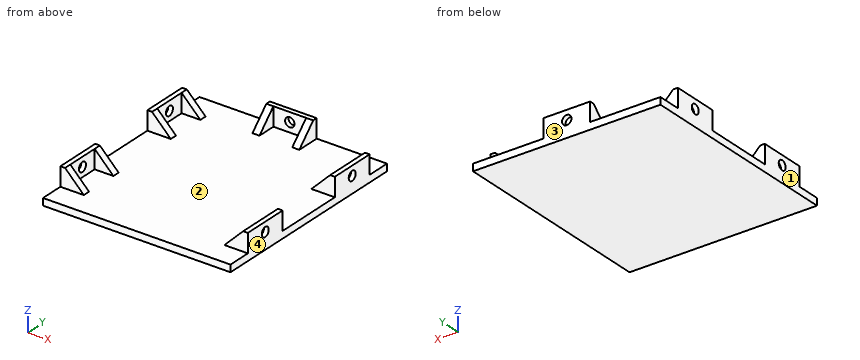
```python
from build123d import *

# Parameters (mm, degrees)
SKETCH1_W               = 80
SKETCH1_H               = 90
BOSS_EXTRUDE1_DEPTH     = 3
BOSS_EXTRUDE2_DEPTH     = 8
CUT_EXTRUDE1_DEPTH      = 114.670576668
SKETCH6_R               = 2
CUT_EXTRUDE3_DEPTH      = 25
MIRROR5_COPY_1_DEPTH    = 8
MIRROR5_COPY_2_DEPTH    = 114.670576668
MIRROR5_COPY_3_SKETCH_R = 2
MIRROR5_COPY_3_DEPTH    = 25
BOSS_EXTRUDE3_DEPTH     = 8
CUT_EXTRUDE2_DEPTH      = 25
SKETCH7_R               = 2
CUT_EXTRUDE4_DEPTH      = 25


with BuildPart() as part:
    # Sketch1 → Boss-Extrude1 (new body)
    with BuildSketch(Plane.XY):
        with Locations((40, 45)):
            Rectangle(SKETCH1_W, SKETCH1_H)
    extrude(amount=BOSS_EXTRUDE1_DEPTH)

    # Sketch2 → Boss-Extrude2 (add)
    with BuildSketch(Plane.XY.offset(3)):
        Polygon((0, 80), (10, 80), (10, 77), (2, 77), (2, 63), (10, 63), (10, 60), (0, 60), align=None)
    boss_extrude2 = extrude(amount=BOSS_EXTRUDE2_DEPTH)

    # Sketch3 → Cut-Extrude1 (cut, through all)
    with BuildSketch(Plane(origin=(0, 80, 0), x_dir=(1, 0, 0), z_dir=(0, 1, 0))):
        Polygon((10, -3), (2, -11), (10, -11), align=None)
    cut_extrude1 = extrude(amount=-CUT_EXTRUDE1_DEPTH, mode=Mode.SUBTRACT)

    # Sketch6 → Cut-Extrude3 (cut)
    with BuildSketch(Plane(origin=(2, 0, 0), x_dir=(0, 0, -1), z_dir=(1, 0, 0))):
        with Locations(Location((-7, 70, 0), (0, 0, 90))):
            Circle(SKETCH6_R)
    cut_extrude3 = extrude(amount=-CUT_EXTRUDE3_DEPTH, mode=Mode.SUBTRACT)

    # Mirror4: Boss-Extrude2, Cut-Extrude1, Cut-Extrude3 across plane
    add(boss_extrude2.mirror(Plane(origin=(40, 0, 0), x_dir=(0, 0, 1), z_dir=(1, 0, 0))))
    add(cut_extrude1.mirror(Plane(origin=(40, 0, 0), x_dir=(0, 0, 1), z_dir=(1, 0, 0))), mode=Mode.SUBTRACT)
    add(cut_extrude3.mirror(Plane(origin=(40, 0, 0), x_dir=(0, 0, 1), z_dir=(1, 0, 0))), mode=Mode.SUBTRACT)

    # Mirror5: Boss-Extrude2, Cut-Extrude1, Cut-Extrude3 across plane
    add(boss_extrude2.mirror(Plane(origin=(0, 45, 0), x_dir=(0, 0, 1), z_dir=(0, -1, 0))))
    add(cut_extrude1.mirror(Plane(origin=(0, 45, 0), x_dir=(0, 0, 1), z_dir=(0, -1, 0))), mode=Mode.SUBTRACT)
    add(cut_extrude3.mirror(Plane(origin=(0, 45, 0), x_dir=(0, 0, 1), z_dir=(0, -1, 0))), mode=Mode.SUBTRACT)

    # Mirror5 copy 1 sketch → Mirror5 copy 1 (add)
    with BuildSketch(Plane(origin=(80, 90, 3), x_dir=(-1, 0, 0), z_dir=(0, 0, 1))):
        Polygon((0, 80), (10, 80), (10, 77), (2, 77), (2, 63), (10, 63), (10, 60), (0, 60), align=None)
    extrude(amount=MIRROR5_COPY_1_DEPTH)

    # Mirror5 copy 2 sketch → Mirror5 copy 2 (cut, through all)
    with BuildSketch(Plane(origin=(80, 10, 0), x_dir=(-1, 0, 0), z_dir=(0, -1, 0))):
        Polygon((10, -3), (2, -11), (10, -11), align=None)
    extrude(amount=-MIRROR5_COPY_2_DEPTH, mode=Mode.SUBTRACT)

    # Mirror5 copy 3 sketch → Mirror5 copy 3 (cut)
    with BuildSketch(Plane(origin=(78, 90, 0), x_dir=(0, 0, -1), z_dir=(-1, 0, 0))):
        with Locations(Location((-7, 70, 0), (0, 0, 90))):
            Circle(MIRROR5_COPY_3_SKETCH_R)
    extrude(amount=-MIRROR5_COPY_3_DEPTH, mode=Mode.SUBTRACT)

    # Sketch4 → Boss-Extrude3 (add)
    with BuildSketch(Plane.XY.offset(3)):
        Polygon((30, 90), (50, 90), (50, 80), (47, 80), (47, 88), (33, 88), (33, 80), (30, 80), align=None)
    extrude(amount=BOSS_EXTRUDE3_DEPTH)

    # Sketch5 → Cut-Extrude2 (cut)
    with BuildSketch(Plane.ZY.offset(-30)):
        Polygon((3, 80), (11, 88), (11, 80), align=None)
    extrude(amount=-CUT_EXTRUDE2_DEPTH, mode=Mode.SUBTRACT)

    # Sketch7 → Cut-Extrude4 (cut)
    with BuildSketch(Plane.XZ.offset(-88)):
        with Locations(Location((40, 7, 0), (0, 0, 270))):
            Circle(SKETCH7_R)
    extrude(amount=-CUT_EXTRUDE4_DEPTH, mode=Mode.SUBTRACT)


solid = part.part
```
CAD build for the part. Positions are in the model's coordinates, mm. Face numbers are marked on the shaded views. Round coordinates to 2 decimals unless told otherwise and drop trailing zeros. Loops run counter-clockwise (first coordinate to the right, second up) from the corner with the lowest first, then second, coordinate; pieces in that order, holes last. Notation, with made-up numbers: M -4,-38.75 L 30,-38.75 A22 ccw 30,-4.75 Z; hole C -36,86 d11. An arc over 180 degrees is marked long. Use a Markdown table: item, result. Add a question column.
(1) Pull direction X, two halves, no side cores. Call the marked faces 1, 2, 3 and 4: +X half, -X half, draft (parallel to the pull), parting line (faces both ways), or undercut.
(2) Drill centre lines: line 1 (Z direction, x = 78.5, y = 20); line 2 (X direction, y = 76, z = 6); line 3 (Z direction, x = 8.5, y = 40). Where is each one in solid material? Low to high.
(3) Cut at B-B (y = 20). Give the cut face in (x, z), and give its area (3 significant figures).
(4) Flat gauge pins, fed straight in: pin 1 (2.5 mm diameter, centred on x = 6.5, z = 7.5, fed in from -Y); pin 2 (12 mm diameter, centred on x = 29, y = 12, fed in from +Z); pin 3 (10 mm diameter, centred on x = 47, y = 79, fed in from +Z). Where does each tip first touch, or does it go through?
(5) Cut at D-D (x = 57.5). Give the cut face in (y, z).
(6) Cut at C-C (z = 7). State how many separate pieces and enclosed holes the cut face has, and give its area (3 significant figures).
(7) Cut at A-A (x = 40). Give the cut face in (y, z), and give its area (3 significant figures).
Geometry says:
| question | item | result |
|---|---|---|
| 1 | face 1 | -X half |
| 1 | face 2 | undercut |
| 1 | face 3 | draft |
| 1 | face 4 | +X half |
| 2 | line 1 | z = 0 to 5, 9 to 11 |
| 2 | line 2 | x = 0 to 2, 78 to 80 |
| 2 | line 3 | z = 0 to 3 |
| 3 | outline | M 0,0 L 80,0 L 80,5 L 78,5 L 78,3 L 2,3 L 2,5 L 0,5 Z; M 0,9 L 2,9 L 2,11 L 0,11 Z; M 78,9 L 80,9 L 80,11 L 78,11 Z |
| 3 | area | 256 mm² |
| 4 | pin 1 | stops at y = 10 |
| 4 | pin 2 | stops at z = 3 |
| 4 | pin 3 | stops at z = 7 |
| 5 | outline | M 0,0 L 90,0 L 90,3 L 0,3 Z |
| 6 | separate pieces | 10 |
| 6 | enclosed holes | 0 |
| 6 | area | 280 mm² |
| 7 | outline | M 0,0 L 90,0 L 90,5 L 88,5 L 88,3 L 0,3 Z; M 88,9 L 90,9 L 90,11 L 88,11 Z |
| 7 | area | 278 mm² |
